from build123d import *

# Parameters (mm, degrees)
BOSS_EXTRUDE1_DEPTH             = 50
SKETCH2_R                       = 25
CUT_EXTRUDE1_DEPTH              = 25
M3X0_5_TAPPED_HOLE1_D           = 2.5
M3X0_5_TAPPED_HOLE1_DEPTH       = 11
M3X0_5_TAPPED_HOLE1_CSINK_D     = 3.05
M3X0_5_TAPPED_HOLE1_CSINK_ANGLE = 90
M3X0_5_TAPPED_HOLE1_TIP         = 0.751075774


with BuildPart() as part:
    # Sketch1 → Boss-Extrude1 (new body)
    with BuildSketch(Plane.XY):
        Polygon((-13, 0), (13, 0), (13, 1), (23, 1), (23, -25), (33, -25), (33, -30), (16, -30), (16, -19), (9, -19), (2, -12), (-2, -12), (-9, -19), (-16, -19), (-16, -30), (-33, -30), (-33, -25), (-23, -25), (-23, 1), (-13, 1), align=None)
    extrude(amount=BOSS_EXTRUDE1_DEPTH)

    # Sketch2 → Cut-Extrude1 (cut)
    with BuildSketch(Plane(origin=(0, 0, 0), x_dir=(-1, 0, 0), z_dir=(0, 0, -1))):
        with Locations((0, 13.2)):
            Circle(SKETCH2_R)
    extrude(amount=-CUT_EXTRUDE1_DEPTH, mode=Mode.SUBTRACT)

    # M3x0.5 Tapped Hole1
    with Locations(Plane(origin=(0, 1, 0), x_dir=(1, 0, 0), z_dir=(0, 1, 0))):
        with Locations((-18, -30), (-18, -45), (18, -30), (18, -45)):
            CounterSinkHole(M3X0_5_TAPPED_HOLE1_D / 2, M3X0_5_TAPPED_HOLE1_CSINK_D / 2, depth=M3X0_5_TAPPED_HOLE1_DEPTH, counter_sink_angle=M3X0_5_TAPPED_HOLE1_CSINK_ANGLE)
            with Locations((0, 0, -(M3X0_5_TAPPED_HOLE1_DEPTH + M3X0_5_TAPPED_HOLE1_TIP / 2))):  # 118° drill point
                Cone(0, M3X0_5_TAPPED_HOLE1_D / 2, M3X0_5_TAPPED_HOLE1_TIP, mode=Mode.SUBTRACT)


solid = part.part
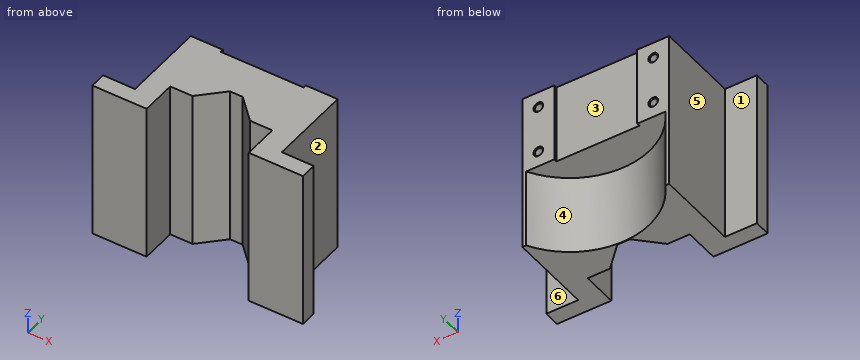
CAD build for the part. Positions are in the model's coordinates, mm. Face numbers are marked on the shaded views. A direction names the side the tool comes from. Coordinates: 2 decimals unless noted, no trailing zeros. Loops run counter-clockwise (first coordinate to the right, second up) from the corner with the lowest first, then second, coordinate; pieces in that order, holes last. Notation, with made-up numbers: (40.5, -22) - (48.5, -22) arc R5 cw to (48.5, -17) - close; hole circle Ø6 at (34, 41.5). An arc over 180 degrees is marked (long way). Write item = value, one per line. Start each with the question number.
Q1. Cut at B-B, the plane z = 7. List the corners of the cut face in (x, y), then the cut area to 3 significant figures.
Q2. Drill centre lines: L1, parallel to Z at x = 18, y = -4.75; L2, parallel to Z at x = -18, y = -1.75; L3, parallel to X at y = -4, z = 45. Where is each one in solid material? Low to high.
Q3. Which spindle directions (+Z, -Z, +X, -X, +Y, -Y) get a long thin tool onto all of the face, cutting with end or side? Do the marked faces 4, 5 and 6. Say none if no direction does.
Q4. Pull direction X, two halves, no side cores. Call the marked faces 1, 2 and 3: pulls with the +X half, pulls with the -X half, needs draft (parallel to the pull), parting line crosses it, or undercut.
Q5. Cut at D-D, the plane x = 27. List the corners of the cut face in (y, z), then the cut area to 3 significant figures.
Q6. Cut at C-C, the plane y = -2. List the corners of the cut face in (x, z), then the cut area to 3 significant figures.
Q7. Flat gauge pins, fed straight in: pin 1 Ø5.5 at (x, z) = (13, 22) entering from -Y; pin 2 Ø2 at (x, z) = (-18, 45) entering from +Y; pin 3 Ø3 at (x, z) = (-27.5, 26.5) entering from +Y; pin 4 Ø1 at (x, y) = (-25, -20.5) entering from -Z. Where does each tip first touch, or does it go through?
Q8. Cut at A-A, the plane y = -16.5. List the corners of the cut face in (x, z), then the cut area to 3 significant figures.
Computed:
q1.outline = (-33, -30) - (-16, -30) - (-16, -19) - (-9, -19) - (-2, -12) - (2, -12) - (9, -19) - (16, -19) - (16, -30) - (33, -30) - (33, -25) - (23, -25) - (23, 1) - (21.82, 1) arc R25 cw to (-21.82, 1) - (-23, 1) - (-23, -25) - (-33, -25) - close
q1.area = 700 mm²
q2.L1 = 0 to 28.75, 31.25 to 43.75, 46.25 to 50
q2.L2 = 25 to 28.75, 31.25 to 43.75, 46.25 to 50
q2.L3 = -23 to -19.25, -16.75 to 16.75, 19.25 to 23
q3.face_4 = -Z, +Y
q3.face_5 = +Z, -Z, -X, +Y
q3.face_6 = +Z, -Z, +X, +Y
q4.face_1 = needs draft
q4.face_2 = pulls with the +X half
q4.face_3 = undercut
q5.outline = (-30, 0) - (-25, 0) - (-25, 50) - (-30, 50) - close
q5.area = 250 mm²
q6.outline = (-23, 0) - (-19.85, 0) - (-19.85, 25) - (19.85, 25) - (19.85, 0) - (23, 0) - (23, 50) - (-23, 50) - close; hole circle Ø2.5 at (-18, 30); hole circle Ø2.5 at (-18, 45); hole circle Ø2.5 at (18, 30); hole circle Ø2.5 at (18, 45)
q6.area = 1,290 mm²
q7.pin_1 = -19
q7.pin_2 = -10.15
q7.pin_3 = -25
q7.pin_4 = through
q8.outline = (-23, 0) - (-6.5, 0) - (-6.5, 50) - (-23, 50) - close; (6.5, 0) - (23, 0) - (23, 50) - (6.5, 50) - close
q8.area = 1,650 mm²
